Verification items for the finished model (mm, model axes). A direction names the side the tool comes from. Give positions to 0.01 mm unless a question says otherwise; leave off trailing zeros. Loops run counter-clockwise (first coordinate to the right, second up) from the corner with the lowest first, then second, coordinate; pieces in that order, holes last. Notation, with made-up numbers: M -5.5,68.5 L 48.5,68.5 A28 cw 48.5,97.5 Z; hole C -36.5,33.25 d6. An arc over 180 degrees is marked long. Answer in a Markdown table with one row per item.
```python
from build123d import *

# Parameters (mm, degrees)
SKETCH1_W                   = 76.2
SKETCH1_H                   = 15.875
BOSS_EXTRUDE1_DEPTH         = 171.45
SKETCH2_W                   = 25.4
SKETCH2_H                   = 15.875
CUT_EXTRUDE1_DEPTH          = 158.75
SKETCH3_W                   = 12.7
SKETCH3_H                   = 15.875
CUT_EXTRUDE2_DEPTH          = 6.35
F_1_4_20_TAPPED_HOLE1_D     = 5.1054
F_1_4_20_TAPPED_HOLE1_DEPTH = 10.8204
F_1_4_20_TAPPED_HOLE1_TIP   = 1.533816902
SKETCH6_R                   = 3.2639
CUT_EXTRUDE3_DEPTH          = 159.75
CUT_EXTRUDE3_DEPTH_BACK     = 13.7


with BuildPart() as part:
    # Sketch1 → Boss-Extrude1 (new body)
    with BuildSketch(Plane.XY):
        Rectangle(SKETCH1_W, SKETCH1_H)
    extrude(amount=BOSS_EXTRUDE1_DEPTH)

    # Sketch2 → Cut-Extrude1 (cut)
    with BuildSketch(Plane.XY.offset(171.45)):
        with Locations((-25.4, 0)):
            Rectangle(SKETCH2_W, SKETCH2_H)
        with Locations((25.4, 0)):
            Rectangle(SKETCH2_W, SKETCH2_H)
    extrude(amount=-CUT_EXTRUDE1_DEPTH, mode=Mode.SUBTRACT)

    # Sketch3 → Cut-Extrude2 (cut)
    with BuildSketch(Plane.XY.offset(171.45)):
        Rectangle(SKETCH3_W, SKETCH3_H)
    extrude(amount=-CUT_EXTRUDE2_DEPTH, mode=Mode.SUBTRACT)

    # 1/4-20 Tapped Hole1
    with Locations(Plane.XY.offset(165.1)):
        with Locations((0, 1.5875)):
            Hole(F_1_4_20_TAPPED_HOLE1_D / 2, depth=F_1_4_20_TAPPED_HOLE1_DEPTH)
            with Locations((0, 0, -(F_1_4_20_TAPPED_HOLE1_DEPTH + F_1_4_20_TAPPED_HOLE1_TIP / 2))):  # 118° drill point
                Cone(0, F_1_4_20_TAPPED_HOLE1_D / 2, F_1_4_20_TAPPED_HOLE1_TIP, mode=Mode.SUBTRACT)

    # Sketch6 → Cut-Extrude3 (cut, two sides)
    with BuildSketch(Plane.XY.offset(12.7)) as cut_extrude3_sk:
        with Locations((-25.4, -1.5875)):
            Circle(SKETCH6_R)
        with Locations((25.4, -1.5875)):
            Circle(SKETCH6_R)
    extrude(amount=CUT_EXTRUDE3_DEPTH, mode=Mode.SUBTRACT)
    extrude(cut_extrude3_sk.sketch, amount=-CUT_EXTRUDE3_DEPTH_BACK, mode=Mode.SUBTRACT)


solid = part.part
```
Item 1: Scan lines: L1, parallel to X at y = -2, z = 8; L2, parallel to Y at x = -25.4, z = 10; L3, parallel to Y at x = 25, z = 6. Record each from-to range of solid material in increasing order. Write a range as [from, to].
Reported:
| item | result |
|---|---|
| L1 | x = [-38.1, -28.64], [-22.16, 22.16], [28.64, 38.1] |
| L2 | y = [-7.94, -4.85], [1.68, 7.94] |
| L3 | y = [-7.94, -4.83], [1.65, 7.94] |
Item 2: Sectioned sample at B-B (x = -27). Record the cut outline in (y, z), and give its area (3 significant figures).
Reported:
| item | result |
|---|---|
| outline | M -7.94,0 L -4.43,0 L -4.43,12.7 L -7.94,12.7 Z; M 1.26,0 L 7.94,0 L 7.94,12.7 L 1.26,12.7 Z |
| area | 129 mm^2 |
Item 3: Sectioned sample at C-C (z = 115). Record the cut outline in (x, y).
Reported:
| item | result |
|---|---|
| outline | M -12.7,-7.94 L 12.7,-7.94 L 12.7,7.94 L -12.7,7.94 Z |
Item 4: Sectioned sample at A-A (x = 25.4). Record the cut outline in (y, z), and give its area (3 significant figures).
Reported:
| item | result |
|---|---|
| outline | M -7.94,0 L -4.85,0 L -4.85,12.7 L -7.94,12.7 Z; M 1.68,0 L 7.94,0 L 7.94,12.7 L 1.68,12.7 Z |
| area | 119 mm^2 |
Item 5: Tool access check on faces 1 (the flat face through (9, 0, 171.45)), 2 (the cylindrical face through (0.553, -0.904, 159.614)), 3 (the flat face through (0, -2, 165.1)), 4 (the flat face through (-26, 2, 12.7)), 5 (the flat face through (25, 2, 12.7)). Record the directions out of +Z, -Z, +X, -X, +Y, -Y that give a thin tool (end or side, any length) a straight path to the whole face; none if there is none.
Reported:
| item | result |
|---|---|
| face 1 | +Z, +X, -X, +Y, -Y |
| face 2 | +Z |
| face 3 | +Z, +Y, -Y |
| face 4 | +Z, -X, +Y, -Y |
| face 5 | +Z, +X, +Y, -Y |
Item 6: Go/stop test with flat-tipped pins: pin 1 (8 mm diameter, centred on x = -21, y = -1, fed in from +Z); pin 2 (3 mm diameter, centred on y = -3, z = 123.5, fed in from +X); pin 3 (4.5 mm diameter, centred on x = 0, y = 1.59, fed in from -Z); pin 4 (6 mm diameter, centred on y = 4.5, z = 51, fed in from -X). Record where each tip stops, or that it passes through.
Reported:
| item | result |
|---|---|
| pin 1 | stops at z = 12.7 |
| pin 2 | stops at x = 12.7 |
| pin 3 | stops at z = 0 |
| pin 4 | stops at x = -12.7 |
Item 7: Release check for a two-part mould opening along X. For faces 6 (the flat face through (-10, 0, 171.45)), 7 (the flat face through (12.7, 0, 93)), 8 (the cylindrical face through (28.513, -0.607, 6.439)) record: released by +X, released by -X, zero draft, split by the parting line, or undercut.
Reported:
| item | result |
|---|---|
| face 6 | zero draft |
| face 7 | released by +X |
| face 8 | undercut |
